Can you work these out from the model? Positions are in its coordinate system, mm. Round coordinates to 2 decimals unless told otherwise and drop trailing zeros. Order: outer loops, then holes, each group sorted by start corner. A loop starts at its lowest first (then second) coordinate and runs counter-clockwise, first axis right, second up. Notation, with made-up numbers: M 55.25,14 L 73.25,14 A17 ccw 73.25,41 Z; hole C 48.25,31 d11. An arc over 180 degrees is marked long. Answer as CSV lines item,"result". Start each with the question number.
from build123d import *

# Parameters (mm, degrees)
BOSS_EXTRU_1_DEPTH      = 175
ESQUISSE2_R             = 3
ENL_V_MAT_EXTRU_1_DEPTH = 4.5
ENL_V_MAT_EXTRU_2_REACH = 177.327
ESQUISSE3_R             = 1.75


with BuildPart() as part:
    # Esquisse1 → Boss.-Extru.1 (new body)
    with BuildSketch(Plane.XY):
        Polygon((-2.287966089, -3.148854962), (9.712033911, -3.148854962), (9.712033911, 1.851145038), (7.712033911, 1.851145038), (7.712033911, 3.051145038), (9.712033911, 3.051145038), (9.712033911, 4.851145038), (-2.287966089, 4.851145038), (-2.287966089, 3.051145038), (-0.287966089, 3.051145038), (-0.287966089, 1.851145038), (-2.287966089, 1.851145038), align=None)
    extrude(amount=BOSS_EXTRU_1_DEPTH)

    # Esquisse2 → Enlèv. mat.-Extru.1 (cut)
    with BuildSketch(Plane(origin=(0, 4.851145038, 0), x_dir=(1, 0, 0), z_dir=(0, 1, 0))):
        with Locations(Location((3.792841972, -162.5, 0), (0, 0, 180))):
            Circle(ESQUISSE2_R)
        with Locations(Location((3.792841972, -137.5, 0), (0, 0, 180))):
            Circle(ESQUISSE2_R)
        with Locations(Location((3.792841972, -112.5, 0), (0, 0, 180))):
            Circle(ESQUISSE2_R)
        with Locations(Location((3.792841972, -87.5, 0), (0, 0, 180))):
            Circle(ESQUISSE2_R)
        with Locations(Location((3.792841972, -62.5, 0), (0, 0, 180))):
            Circle(ESQUISSE2_R)
        with Locations(Location((3.792841972, -37.5, 0), (0, 0, 180))):
            Circle(ESQUISSE2_R)
        with Locations(Location((3.792841972, -12.5, 0), (0, 0, 180))):
            Circle(ESQUISSE2_R)
    extrude(amount=-ENL_V_MAT_EXTRU_1_DEPTH, mode=Mode.SUBTRACT)

    # Esquisse3 → Enlèv. mat.-Extru.2 (cut, up to next)
    with BuildSketch(Plane(origin=(0, 0.351145038, 0), x_dir=(1, 0, 0), z_dir=(0, 1, 0)), mode=Mode.PRIVATE) as enl_v_mat_extru_2_sk1:
        with Locations(Location((3.792841972, -162.5, 0), (0, 0, 180))):
            Circle(ESQUISSE3_R)
    enl_v_mat_extru_2_tool1 = extrude(enl_v_mat_extru_2_sk1.sketch, amount=-ENL_V_MAT_EXTRU_2_REACH, mode=Mode.PRIVATE) & part.part
    # Esquisse3 → Enlèv. mat.-Extru.2 (cut, up to next)
    with BuildSketch(Plane(origin=(0, 0.351145038, 0), x_dir=(1, 0, 0), z_dir=(0, 1, 0)), mode=Mode.PRIVATE) as enl_v_mat_extru_2_sk2:
        with Locations(Location((3.792841972, -137.5, 0), (0, 0, 180))):
            Circle(ESQUISSE3_R)
    enl_v_mat_extru_2_tool2 = extrude(enl_v_mat_extru_2_sk2.sketch, amount=-ENL_V_MAT_EXTRU_2_REACH, mode=Mode.PRIVATE) & part.part
    # Esquisse3 → Enlèv. mat.-Extru.2 (cut, up to next)
    with BuildSketch(Plane(origin=(0, 0.351145038, 0), x_dir=(1, 0, 0), z_dir=(0, 1, 0)), mode=Mode.PRIVATE) as enl_v_mat_extru_2_sk3:
        with Locations(Location((3.792841972, -112.5, 0), (0, 0, 180))):
            Circle(ESQUISSE3_R)
    enl_v_mat_extru_2_tool3 = extrude(enl_v_mat_extru_2_sk3.sketch, amount=-ENL_V_MAT_EXTRU_2_REACH, mode=Mode.PRIVATE) & part.part
    # Esquisse3 → Enlèv. mat.-Extru.2 (cut, up to next)
    with BuildSketch(Plane(origin=(0, 0.351145038, 0), x_dir=(1, 0, 0), z_dir=(0, 1, 0)), mode=Mode.PRIVATE) as enl_v_mat_extru_2_sk4:
        with Locations(Location((3.792841972, -87.5, 0), (0, 0, 180))):
            Circle(ESQUISSE3_R)
    enl_v_mat_extru_2_tool4 = extrude(enl_v_mat_extru_2_sk4.sketch, amount=-ENL_V_MAT_EXTRU_2_REACH, mode=Mode.PRIVATE) & part.part
    # Esquisse3 → Enlèv. mat.-Extru.2 (cut, up to next)
    with BuildSketch(Plane(origin=(0, 0.351145038, 0), x_dir=(1, 0, 0), z_dir=(0, 1, 0)), mode=Mode.PRIVATE) as enl_v_mat_extru_2_sk5:
        with Locations(Location((3.792841972, -62.5, 0), (0, 0, 180))):
            Circle(ESQUISSE3_R)
    enl_v_mat_extru_2_tool5 = extrude(enl_v_mat_extru_2_sk5.sketch, amount=-ENL_V_MAT_EXTRU_2_REACH, mode=Mode.PRIVATE) & part.part
    # Esquisse3 → Enlèv. mat.-Extru.2 (cut, up to next)
    with BuildSketch(Plane(origin=(0, 0.351145038, 0), x_dir=(1, 0, 0), z_dir=(0, 1, 0)), mode=Mode.PRIVATE) as enl_v_mat_extru_2_sk6:
        with Locations(Location((3.792841972, -37.5, 0), (0, 0, 180))):
            Circle(ESQUISSE3_R)
    enl_v_mat_extru_2_tool6 = extrude(enl_v_mat_extru_2_sk6.sketch, amount=-ENL_V_MAT_EXTRU_2_REACH, mode=Mode.PRIVATE) & part.part
    # Esquisse3 → Enlèv. mat.-Extru.2 (cut, up to next)
    with BuildSketch(Plane(origin=(0, 0.351145038, 0), x_dir=(1, 0, 0), z_dir=(0, 1, 0)), mode=Mode.PRIVATE) as enl_v_mat_extru_2_sk7:
        with Locations(Location((3.792841972, -12.5, 0), (0, 0, 180))):
            Circle(ESQUISSE3_R)
    enl_v_mat_extru_2_tool7 = extrude(enl_v_mat_extru_2_sk7.sketch, amount=-ENL_V_MAT_EXTRU_2_REACH, mode=Mode.PRIVATE) & part.part
    add(enl_v_mat_extru_2_tool1.solids().sort_by_distance((3.792842, 0.351145, 162.5))[0], mode=Mode.SUBTRACT)
    add(enl_v_mat_extru_2_tool2.solids().sort_by_distance((3.792842, 0.351145, 137.5))[0], mode=Mode.SUBTRACT)
    add(enl_v_mat_extru_2_tool3.solids().sort_by_distance((3.792842, 0.351145, 112.5))[0], mode=Mode.SUBTRACT)
    add(enl_v_mat_extru_2_tool4.solids().sort_by_distance((3.792842, 0.351145, 87.5))[0], mode=Mode.SUBTRACT)
    add(enl_v_mat_extru_2_tool5.solids().sort_by_distance((3.792842, 0.351145, 62.5))[0], mode=Mode.SUBTRACT)
    add(enl_v_mat_extru_2_tool6.solids().sort_by_distance((3.792842, 0.351145, 37.5))[0], mode=Mode.SUBTRACT)
    add(enl_v_mat_extru_2_tool7.solids().sort_by_distance((3.792842, 0.351145, 12.5))[0], mode=Mode.SUBTRACT)


solid = part.part
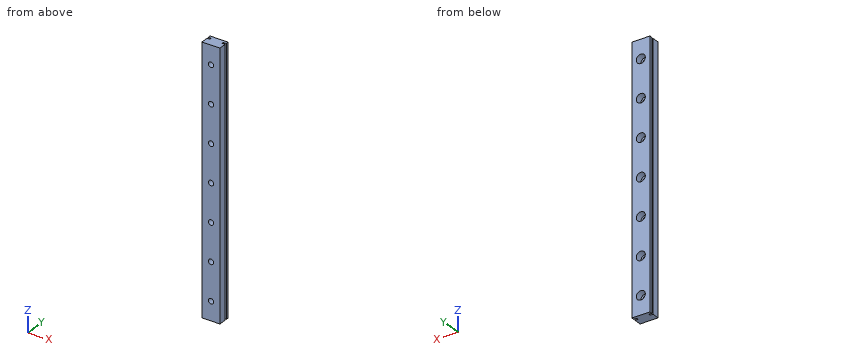
(1) I'm going to push flat-ended pins straight in: P1, Ø5.5, axis at x = 3.79, z = 62.5, coming from the +Y side; P2, Ø3, axis at x = 3.79, z = 112.5, coming from the -Y side. Where does each tip first touch, or does it pass through?
(2) I want a section at A-A on y = -1.75. Write out the boundary of the cut face in (x, z).
(3) I want a section at B-B on z = 12.5. Write out the boundary of the cut face in (x, y), and give its area (4 significant figures).
(4) If I drill on line 1 along X through (y, z) = (-0.75, 112.5); line 2 along Y through (x, z) = (9, 156); line 3 along X through (y, z) = (2.5, 54), over which ranges is the centre line in solid material (lowest first)?
(5) I want a section at C-C on z = 127. Write out the boundary of the cut face in (x, y).
(6) I want a section at D-D on x = 4. Count the separate pieces of the cut face and the enclosed holes in it, and give its area (3 significant figures).
From the geometry:
1,P1,"y = 0.35"
1,P2,"through"
2,outline,"M -2.29,0 L 9.71,0 L 9.71,175 L -2.29,175 Z; hole C 3.79,12.5 d3.5; hole C 3.79,37.5 d3.5; hole C 3.79,62.5 d3.5; hole C 3.79,87.5 d3.5; hole C 3.79,112.5 d3.5; hole C 3.79,137.5 d3.5; hole C 3.79,162.5 d3.5"
3,outline,"M -2.29,-3.15 L 2.04,-3.15 L 2.04,0.35 L 0.79,0.35 L 0.79,4.85 L -2.29,4.85 L -2.29,3.05 L -0.29,3.05 L -0.29,1.85 L -2.29,1.85 Z; M 5.54,-3.15 L 9.71,-3.15 L 9.71,1.85 L 7.71,1.85 L 7.71,3.05 L 9.71,3.05 L 9.71,4.85 L 6.79,4.85 L 6.79,0.35 L 5.54,0.35 Z"
3,area,"51.95 mm²"
4,line 1,"-2.29 to 2.04, 5.54 to 9.71"
4,line 2,"-3.15 to 1.85, 3.05 to 4.85"
4,line 3,"-0.29 to 7.71"
5,outline,"M -2.29,-3.15 L 9.71,-3.15 L 9.71,1.85 L 7.71,1.85 L 7.71,3.05 L 9.71,3.05 L 9.71,4.85 L -2.29,4.85 L -2.29,3.05 L -0.29,3.05 L -0.29,1.85 L -2.29,1.85 Z"
6,separate pieces,"8"
6,enclosed holes,"0"
6,area,"1,130 mm²"
